Can you work these out from the drawing? Everything is in mm from the part's minimum corner. Coordinates: 2 decimals unless noted, no trailing zeros. Write each loop counter-clockwise with the first axis right and the second up, starting at its lowest first coordinate (ties: lowest second). Pieces come first, ordered by that corner, then holes. Notation, with made-up numbers: (31.25, 28) -> (47.25, 28) arc R8 ccw to (47.25, 37) -> close; hole circle Ø1 at (81.5, 26). An arc over 180 degrees is marked (long way). Use a Markdown table: item, result. Add a question column.
Item 1: Imagine slicing it at C-C, the plane y = 1.1. Write out the boundary of the cut face in (x, z).
Item 2: Will these pins go through, and if not, where does the flat tip stop? pin 1 Ø4.5 at (x, z) = (12.7, 12.7) entering from -Y; pin 2 Ø4.5 at (x, z) = (12.7, 31.75) entering from +Y.
Item 3: Imagine slicing it at B-B, the plane x = 12.7. Write out the boundary of the cut face in (y, z), and give its area (3 significant figures).
Item 4: Imagine slicing it at D-D, the plane x = 16. Write out the boundary of the cut face in (y, z).
Item 5: If I drill on line 1 along Z through (x, y) = (12.5, 0.35); line 2 along X through (y, z) = (1.5, 12.7); line 3 along Z through (x, y) = (11, 0.7), over which ranges is the centre line in solid material (lowest first)? Write a range as from..to.
Item 6: Imagine slicing it at A-A, the plane z = 12.7. Write out the boundary of the cut face in (x, y), and give its area (3 significant figures).
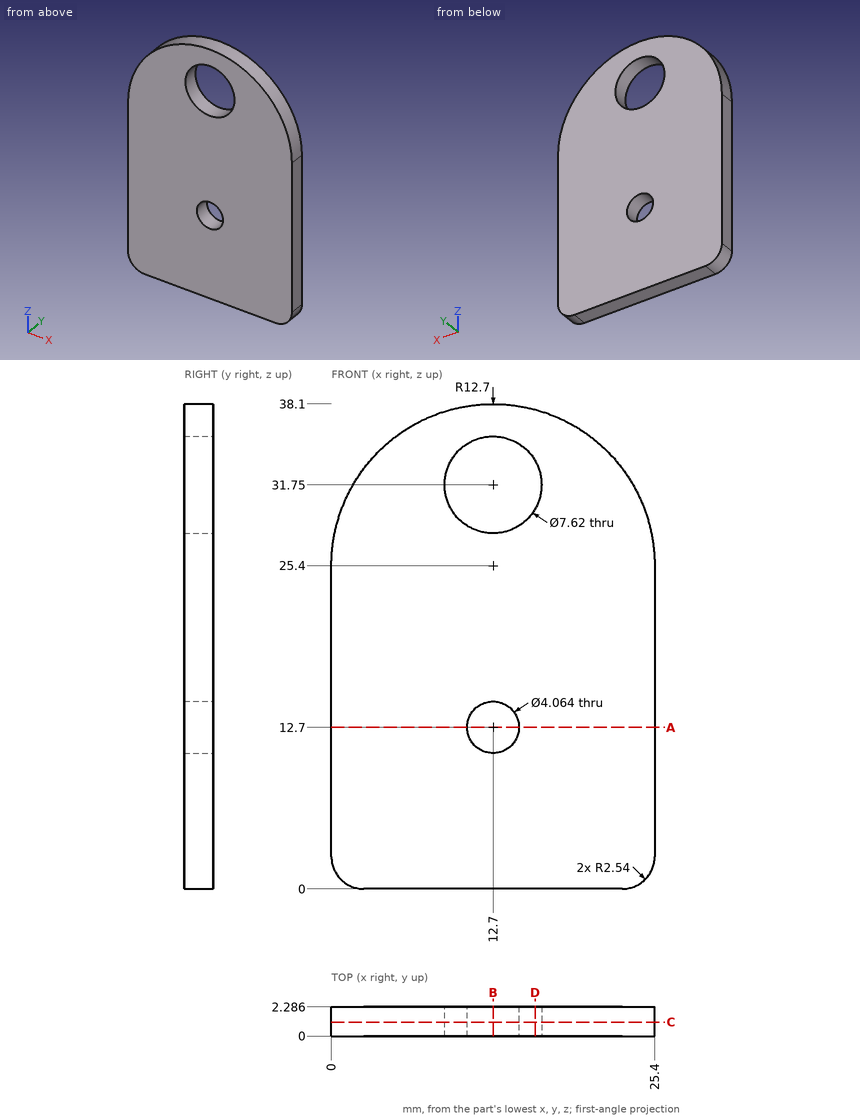
Ans:
| question | item | result |
|---|---|---|
| 1 | outline | (0, 2.54) arc R2.54 ccw to (2.54, 0) -> (22.86, 0) arc R2.54 ccw to (25.4, 2.54) -> (25.4, 25.4) arc R12.7 ccw to (0, 25.4) -> close; hole circle Ø7.62 at (12.7, 31.75); hole circle Ø4.06 at (12.7, 12.7) |
| 2 | pin 1 | stops at y = 0 |
| 2 | pin 2 | passes through |
| 3 | outline | (0, 0) -> (2.29, 0) -> (2.29, 10.67) -> (0, 10.67) -> close; (0, 14.73) -> (2.29, 14.73) -> (2.29, 27.94) -> (0, 27.94) -> close; (0, 35.56) -> (2.29, 35.56) -> (2.29, 38.1) -> (0, 38.1) -> close |
| 3 | area | 60.4 mm^2 |
| 4 | outline | (0, 0) -> (2.29, 0) -> (2.29, 29.85) -> (0, 29.85) -> close; (0, 33.65) -> (2.29, 33.65) -> (2.29, 37.66) -> (0, 37.66) -> close |
| 5 | line 1 | z = 0..10.68, 14.72..27.95, 35.55..38.1 |
| 5 | line 2 | x = 0..10.67, 14.73..25.4 |
| 5 | line 3 | z = 0..11.59, 13.81..28.34, 35.16..37.99 |
| 6 | outline | (0, 0) -> (10.67, 0) -> (10.67, 2.29) -> (0, 2.29) -> close; (14.73, 0) -> (25.4, 0) -> (25.4, 2.29) -> (14.73, 2.29) -> close |
| 6 | area | 48.8 mm^2 |
